Source: CAD feature listing. Evaluate the final solid. Frame: model axes, mm. A direction names the side the tool comes from. Coordinates: 2 decimals unless noted, no trailing zeros. Order: outer loops, then holes, each group sorted by start corner. A loop starts at its lowest first (then second) coordinate and runs counter-clockwise, first axis right, second up.
```python
from build123d import *

# Parameters (mm, degrees)
SKETCH2_W          = 5.6237504
SKETCH2_H          = 5.000603239
CUT_EXTRUDE1_DEPTH = 50


with BuildPart() as part:
    # Sketch1 → Revolve-Thin1 (revolve)
    with BuildSketch(Plane.XY, mode=Mode.PRIVATE) as revolve_thin1_sk:
        Polygon((-35, -30), (-20, -30), (-20, -40), (-35, -40), (-35, -50), (-10, -50), (-10, -20), (-35, -20), align=None)
    revolve(revolve_thin1_sk.sketch.rotate(Axis((-102.944705745, -57.920177064, 0), (1, 0, 0)), 90), axis=Axis((-102.944705745, -57.920177064, 0), (1, 0, 0)))

    # Sketch2 → Cut-Extrude1 (cut)
    with BuildSketch(Plane.ZY.offset(35)):
        with Locations((0, -65.840354128)):
            Rectangle(SKETCH2_W, SKETCH2_H)
    extrude(amount=-CUT_EXTRUDE1_DEPTH, mode=Mode.SUBTRACT)


solid = part.part
```
1. Section query B-B on x = -33.5. Return loops of the section in (y, z).
Findings:
outline: circle Ø75.84 at (-57.92, 0); circle Ø35.84 at (-57.92, 0); hole circle Ø55.84 at (-57.92, 0); hole (-68.34, -2.81) - (-65.32, -2.81) arc R7.92 ccw (long way) to (-65.32, 2.81) - (-68.34, 2.81) - close
2. Section query D-D on x = -18. Return loops of the section in (y, z), plus the area to 3 significant figures.
Findings:
outline: circle Ø75.84 at (-57.92, 0); hole (-68.34, -2.81) - (-65.32, -2.81) arc R7.92 ccw (long way) to (-65.32, 2.81) - (-68.34, 2.81) - close
area: 4,310 mm2
3. Section query C-C on y = -82. Return loops of the section in (x, z).
Findings:
outline: (-35, -29.29) - (-10, -29.29) - (-10, 29.29) - (-35, 29.29) - (-35, 14.13) - (-20, 14.13) - (-20, -14.13) - (-35, -14.13) - close
4. Access query for faces 1 (the face through (-20, -39.7, -0.4)), 2 (the face through (-35, -50, 4)), 3 (the face through (-23, -67, -2.812)). Directions: +Z, -Z, +X, -X, +Y, -Y. A direction counts if a zero-diameter tool reaches every point of the face in a straight line with its end or side. Return the directions, or none.
Findings:
face 1: -X
face 2: +Z, -Z, -X, +Y, -Y
face 3: +X, -X
5. Ray query, line 1 (Z direction, x = -31, y = -58); line 2 (Y direction, x = -29.75, z = -8.5); line 3 (Y direction, x = -27.75, z = -5). Return the intervals inside material, ascending.
Findings:
line 1: z = -37.92 to -27.92, -17.92 to -7.92, 7.92 to 17.92, 27.92 to 37.92
line 2: y = -94.88 to -84.52, -73.7 to -42.14, -31.33 to -20.96
line 3: y = -95.51 to -85.39, -75.13 to -64.06, -51.78 to -40.71, -30.45 to -20.33
6. Draft query along Y for faces 4 (the face through (-10, -58, 9)), 5 (the face through (-22.675, -95.518, -4.936)), 6 (the face through (-27.395, -30.664, -6.053)). Return one class per face: released by +Y, released by -Y, zero draft, split by the parting line, or undercut.
Findings:
face 4: zero draft
face 5: split by the parting line
face 6: undercut
7. Section query A-A on z = 0. Return loops of the section in (x, y).
Findings:
outline: (-35, -95.84) - (-10, -95.84) - (-10, -68.34) - (-35, -68.34) - (-35, -75.84) - (-20, -75.84) - (-20, -85.84) - (-35, -85.84) - close; (-35, -50) - (-10, -50) - (-10, -20) - (-35, -20) - (-35, -30) - (-20, -30) - (-20, -40) - (-35, -40) - close
8. Pin query (flat end, axial travel): P1, Ø1, axis at x = -20.5, y = -40.5, coming from the +Z side; P2, Ø1, axis at x = -27, z = -7.5, coming from the -Y side; P3, Ø1.5, axis at x = -16, y = -41, coming from the +Z side. Return the tip coordinate at first contact, or that it passes through.
Findings:
P1: stops at z = 33.94
P2: stops at y = -95.19
P3: stops at z = 34.3
